```python
from build123d import *

# Parameters (mm, degrees)
BOSS_EXTRUDE1_DEPTH = 6.35
CUT_EXTRUDE5_DEPTH  = 1432.25665609
CUT_EXTRUDE6_DEPTH  = 721.614
SKETCH19_W          = 812.8
SKETCH19_H          = 6.35
BOSS_EXTRUDE8_DEPTH = 3.175
SKETCH20_W          = 812.8
SKETCH20_H          = 6.35
BOSS_EXTRUDE9_DEPTH = 38.1
FILLET1_R           = 6.35
FILLET2_R           = 6.35
CUT_EXTRUDE7_REACH  = 8.35
SKETCH22_R          = 3.175


with BuildPart() as part:
    # Sketch1 → Boss-Extrude1 (new body)
    with BuildSketch(Plane.XY):
        Polygon((-812.8, 0), (0, 0), (609.6, -165.1), (304.8, -165.1), align=None)
    extrude(amount=BOSS_EXTRUDE1_DEPTH)

    # Sketch17 → Cut-Extrude5 (cut, through all)
    with BuildSketch(Plane(origin=(-795.440818906, 117.508302793, 0), x_dir=(0, 0, -1), z_dir=(-0.989263736, 0.146141234, 0))):
        Polygon((-3.175, 118.7835948), (-6.35, 109.011949569), (-6.35, 209.992544036), (0, 209.992544036), (0, 109.011949569), align=None)
    extrude(amount=-CUT_EXTRUDE5_DEPTH, mode=Mode.SUBTRACT)

    # Sketch18 → Cut-Extrude6 (cut)
    with BuildSketch(Plane(origin=(609.6, -165.1, 0), x_dir=(0, 0, -1), z_dir=(0.965226372, -0.261415476, 0))):
        Polygon((-3.175, 0), (-6.35, -9.771645231), (-6.35, 0.882856688), (0, 0.882856688), (0, -9.771645231), align=None)
    extrude(amount=-CUT_EXTRUDE6_DEPTH, mode=Mode.SUBTRACT)

    # Sketch19 → Boss-Extrude8 (add)
    with BuildSketch(Plane(origin=(0, 0, 0), x_dir=(1, 0, 0), z_dir=(0, 1, 0))):
        with Locations((-406.4, -3.175)):
            Rectangle(SKETCH19_W, SKETCH19_H)
    extrude(amount=BOSS_EXTRUDE8_DEPTH)

    # Sketch20 → Boss-Extrude9 (add)
    with BuildSketch(Plane(origin=(0, 3.175, 0), x_dir=(1, 0, 0), z_dir=(0, 1, 0))):
        with Locations((-406.4, -3.175)):
            Rectangle(SKETCH20_W, SKETCH20_H)
    extrude(amount=BOSS_EXTRUDE9_DEPTH)

    # Fillet1
    fillet1_edges = [part.edges().sort_by_distance(p)[0] for p in [
        (0, 41.275, 3.175),
    ]]
    fillet(fillet1_edges, radius=FILLET1_R)

    # Fillet2
    fillet2_edges = [part.edges().sort_by_distance(p)[0] for p in [
        (-812.8, 41.275, 3.175),
    ]]
    fillet(fillet2_edges, radius=FILLET2_R)

    # Sketch22 → Cut-Extrude7 (cut, up to next)
    with BuildSketch(Plane(origin=(0, 0, 0), x_dir=(-1, 0, 0), z_dir=(0, 0, -1)), mode=Mode.PRIVATE) as cut_extrude7_sk1:
        with Locations((149.225, 25.4)):
            Circle(SKETCH22_R)
    cut_extrude7_tool1 = extrude(cut_extrude7_sk1.sketch, amount=-CUT_EXTRUDE7_REACH, mode=Mode.PRIVATE) & part.part
    add(cut_extrude7_tool1.solids().sort_by_distance((-149.225, 25.4, 0))[0], mode=Mode.SUBTRACT)
    # Sketch22 → Cut-Extrude7 (cut, up to next)
    with BuildSketch(Plane(origin=(0, 0, 0), x_dir=(-1, 0, 0), z_dir=(0, 0, -1)), mode=Mode.PRIVATE) as cut_extrude7_sk2:
        with Locations((796.925, 25.4)):
            Circle(SKETCH22_R)
    cut_extrude7_tool2 = extrude(cut_extrude7_sk2.sketch, amount=-CUT_EXTRUDE7_REACH, mode=Mode.PRIVATE) & part.part
    add(cut_extrude7_tool2.solids().sort_by_distance((-796.925, 25.4, 0))[0], mode=Mode.SUBTRACT)
    # Sketch22 → Cut-Extrude7 (cut, up to next)
    with BuildSketch(Plane(origin=(0, 0, 0), x_dir=(-1, 0, 0), z_dir=(0, 0, -1)), mode=Mode.PRIVATE) as cut_extrude7_sk3:
        with Locations((663.575, 25.4)):
            Circle(SKETCH22_R)
    cut_extrude7_tool3 = extrude(cut_extrude7_sk3.sketch, amount=-CUT_EXTRUDE7_REACH, mode=Mode.PRIVATE) & part.part
    add(cut_extrude7_tool3.solids().sort_by_distance((-663.575, 25.4, 0))[0], mode=Mode.SUBTRACT)
    # Sketch22 → Cut-Extrude7 (cut, up to next)
    with BuildSketch(Plane(origin=(0, 0, 0), x_dir=(-1, 0, 0), z_dir=(0, 0, -1)), mode=Mode.PRIVATE) as cut_extrude7_sk4:
        with Locations((581.025, 25.4)):
            Circle(SKETCH22_R)
    cut_extrude7_tool4 = extrude(cut_extrude7_sk4.sketch, amount=-CUT_EXTRUDE7_REACH, mode=Mode.PRIVATE) & part.part
    add(cut_extrude7_tool4.solids().sort_by_distance((-581.025, 25.4, 0))[0], mode=Mode.SUBTRACT)
    # Sketch22 → Cut-Extrude7 (cut, up to next)
    with BuildSketch(Plane(origin=(0, 0, 0), x_dir=(-1, 0, 0), z_dir=(0, 0, -1)), mode=Mode.PRIVATE) as cut_extrude7_sk5:
        with Locations((447.675, 25.4)):
            Circle(SKETCH22_R)
    cut_extrude7_tool5 = extrude(cut_extrude7_sk5.sketch, amount=-CUT_EXTRUDE7_REACH, mode=Mode.PRIVATE) & part.part
    add(cut_extrude7_tool5.solids().sort_by_distance((-447.675, 25.4, 0))[0], mode=Mode.SUBTRACT)
    # Sketch22 → Cut-Extrude7 (cut, up to next)
    with BuildSketch(Plane(origin=(0, 0, 0), x_dir=(-1, 0, 0), z_dir=(0, 0, -1)), mode=Mode.PRIVATE) as cut_extrude7_sk6:
        with Locations((365.125, 25.4)):
            Circle(SKETCH22_R)
    cut_extrude7_tool6 = extrude(cut_extrude7_sk6.sketch, amount=-CUT_EXTRUDE7_REACH, mode=Mode.PRIVATE) & part.part
    add(cut_extrude7_tool6.solids().sort_by_distance((-365.125, 25.4, 0))[0], mode=Mode.SUBTRACT)
    # Sketch22 → Cut-Extrude7 (cut, up to next)
    with BuildSketch(Plane(origin=(0, 0, 0), x_dir=(-1, 0, 0), z_dir=(0, 0, -1)), mode=Mode.PRIVATE) as cut_extrude7_sk7:
        with Locations((231.775, 25.4)):
            Circle(SKETCH22_R)
    cut_extrude7_tool7 = extrude(cut_extrude7_sk7.sketch, amount=-CUT_EXTRUDE7_REACH, mode=Mode.PRIVATE) & part.part
    add(cut_extrude7_tool7.solids().sort_by_distance((-231.775, 25.4, 0))[0], mode=Mode.SUBTRACT)
    # Sketch22 → Cut-Extrude7 (cut, up to next)
    with BuildSketch(Plane(origin=(0, 0, 0), x_dir=(-1, 0, 0), z_dir=(0, 0, -1)), mode=Mode.PRIVATE) as cut_extrude7_sk8:
        with Locations((15.875, 25.4)):
            Circle(SKETCH22_R)
    cut_extrude7_tool8 = extrude(cut_extrude7_sk8.sketch, amount=-CUT_EXTRUDE7_REACH, mode=Mode.PRIVATE) & part.part
    add(cut_extrude7_tool8.solids().sort_by_distance((-15.875, 25.4, 0))[0], mode=Mode.SUBTRACT)


solid = part.part
```
Check sheet for the modelled part. Datum: model origin and axes. Units: mm. Round coordinates to 2 decimals unless told otherwise and drop trailing zeros. Loops run counter-clockwise (first coordinate to the right, second up) from the corner with the lowest first, then second, coordinate; pieces in that order, holes last. Notation, with made-up numbers: (56.25, -9.75) - (89.25, -9.75) arc R9 cw to (89.25, 2.25) - close; hole circle Ø1 at (50.25, 18). An arc over 180 degrees is marked (long way). Write item = value, one per line. Start each with the question number.
Q1. Section check B-B (y = -25). Record the boundary of the cut face in (x, z) (3 decimals).
Q2. Section check D-D (x = 462.5). Record the boundary of the cut face in (y, z) (3 decimals), plus the area to 3 significant figures.
Q3. Thickness scan on L1, parallel to Z at x = 283, y = -78.5; L2, parallel to Z at x = -731, y = -7. Record the ranges inside material, lowest first.
Q4. Section check A-A (z = 5.25). Count the separate pieces of the cut face and the enclosed holes in it, plus the area to 3 significant figures.
Q5. Depth check by flat-ended pin: P1, Ø3.5, axis at x = -767.5, z = 4.5, coming from the -Y side; P2, Ø3.5, axis at x = -9.5, z = 4.5, coming from the -Y side; P3, Ø8.5, axis at x = -365.125, y = 25.4, coming from the -Z side; P4, Ø5.5, axis at x = -231.775, y = 25.4, coming from the +Z side. Enter the tip coordinate at first touch or a pass-through.
Q6. Section check C-C (x = 217). Record the boundary of the cut face in (y, z) (3 decimals), plus the area to 3 significant figures.
Derived:
q1.outline = (-643.569, 3.175) - (-576.705, 0) - (54.928, 0) - (92.308, 3.175) - (54.928, 6.35) - (-576.705, 6.35) - close
q2.outline = (-165.1, 0) - (-135.384, 0) - (-125.26, 3.175) - (-135.384, 6.35) - (-165.1, 6.35) - close
q2.area = 221 mm^2
q3.L1 = 2.59 to 3.76
q3.L2 = 1.54 to 4.81
q4.separate_pieces = 1
q4.enclosed_holes = 8
q4.area = 114,000 mm^2
q5.P1 = -6.86
q5.P2 = -118.84
q5.P3 = 0
q5.P4 = through
q6.outline = (-152.13, 3.175) - (-142.252, 0) - (-68.895, 0) - (-58.771, 3.175) - (-68.895, 6.35) - (-142.252, 6.35) - close
q6.area = 529 mm^2
